Geometry: final body of the model. Coordinates: model frame, mm. A direction names the side the tool comes from. Give positions to 0.01 mm unless a question says otherwise; leave off trailing zeros. Order: outer loops, then holes, each group sorted by start corner. A loop starts at its lowest first (then second) coordinate and runs counter-clockwise, first axis right, second up. Notation, with made-up numbers: (-19, 36) - (7, 36) arc R26 cw to (7, 58) - close; hole circle Ø11 at (8.5, 11). An arc over 180 degrees is marked (long way). Use one line per item in the form item = value.
from build123d import *

# Parameters (mm, degrees)
SKETCH_1_W             = 300
SKETCH_1_H             = 300
EXTRUDE_2_DEPTH        = 5
SKETCH_4_W             = 45
SKETCH_4_H             = 60
CUT_EXTRUDE_3_DEPTH    = 5
SKETCH_5_OUTSIDE_W     = 386.858
SKETCH_5_OUTSIDE_H     = 386.858
SKETCH_5_OUTSIDE_W_2   = 250
SKETCH_5_OUTSIDE_H_2   = 300
CUT_EXTRUDE_4_DEPTH    = 5
SKETCH_6_R             = 1.75
SKETCH_6_R_2           = 1.25
CUT_EXTRUDE_5_DEPTH    = 5
SKETCH_7_W             = 50
SKETCH_7_H             = 70
CUT_EXTRUDE_6_DEPTH    = 10
SKETCH_8_W             = 30
SKETCH_8_H             = 24.494897428
SKETCH_8_W_2           = 120
SKETCH_8_H_2           = 10
CUT_EXTRUDE_7_DEPTH    = 10
FILLET_1_R             = 3
HOLE_WIZARD_M3_1_D     = 2.5
HOLE_WIZARD_M3_1_DEPTH = 10
HOLE_WIZARD_M3_1_TIP   = 0.751075774


with BuildPart() as part:
    # 草图1 → 凸台-拉伸2 (new body)
    with BuildSketch(Plane.XY):
        Rectangle(SKETCH_1_W, SKETCH_1_H)
    extrude(amount=EXTRUDE_2_DEPTH)

    # 草图4 → 切除-拉伸3 (cut)
    with BuildSketch(Plane.XY.offset(5)):
        with Locations((0, 120)):
            Rectangle(SKETCH_4_W, SKETCH_4_H)
    extrude(amount=-CUT_EXTRUDE_3_DEPTH, mode=Mode.SUBTRACT)

    # 草图5 outside → 切除-拉伸4 (cut)
    with BuildSketch(Plane.XY.offset(5)):
        Rectangle(SKETCH_5_OUTSIDE_W, SKETCH_5_OUTSIDE_H)
        Rectangle(SKETCH_5_OUTSIDE_W_2, SKETCH_5_OUTSIDE_H_2, mode=Mode.SUBTRACT)
    extrude(amount=-CUT_EXTRUDE_4_DEPTH, mode=Mode.SUBTRACT)

    # 草图6 → 切除-拉伸5 (cut)
    with BuildSketch(Plane.XY.offset(5)):
        with Locations((-85, 110)):
            Circle(SKETCH_6_R)
        with Locations((-61, 110)):
            Circle(SKETCH_6_R)
        with Locations((-61, 80)):
            Circle(SKETCH_6_R)
        with Locations((-85, 80)):
            Circle(SKETCH_6_R)
        with Locations((85, 80)):
            Circle(SKETCH_6_R)
        with Locations((61, 80)):
            Circle(SKETCH_6_R)
        with Locations((61, 110)):
            Circle(SKETCH_6_R)
        with Locations((85, 110)):
            Circle(SKETCH_6_R)
        with Locations((-47, -100)):
            Circle(SKETCH_6_R_2)
        with Locations((-47, -44)):
            Circle(SKETCH_6_R_2)
        with Locations((47, -44)):
            Circle(SKETCH_6_R_2)
        with Locations((47, -100)):
            Circle(SKETCH_6_R_2)
        with Locations((-35, 105)):
            Circle(SKETCH_6_R)
        with Locations((-35, 85)):
            Circle(SKETCH_6_R)
        with Locations((35, 85)):
            Circle(SKETCH_6_R)
        with Locations((35, 105)):
            Circle(SKETCH_6_R)
    extrude(amount=-CUT_EXTRUDE_5_DEPTH, mode=Mode.SUBTRACT)

    # 草图7 → 切除-拉伸6 (cut)
    with BuildSketch(Plane.XY.offset(5)):
        with Locations((-125, 95)):
            Rectangle(SKETCH_7_W, SKETCH_7_H)
        with Locations((125, 95)):
            Rectangle(SKETCH_7_W, SKETCH_7_H)
    extrude(amount=-CUT_EXTRUDE_6_DEPTH, mode=Mode.SUBTRACT)

    # 草图8 → 切除-拉伸7 (cut)
    with BuildSketch(Plane.XY.offset(5)):
        Polygon((-125, 130), (-73.75, 150), (-125, 150), align=None)
        Polygon((125, 130), (73.75, 150), (125, 150), align=None)
        with BuildLine():
            Line((75, -150), (125, -150))
            Line((125, -150), (125, 60))
            Line((125, 60), (105, 60))
            Line((105, 60), (105, -134.641016151))
            ThreePointArc((105, -134.641016151), (103.660254038, -139.641016151), (100, -143.301270189))
            ThreePointArc((100, -143.301270189), (87.940952255, -148.296291314), (75, -150))
        make_face()
        with Locations((-55, -137.752551286)):
            Rectangle(SKETCH_8_W, SKETCH_8_H)
        with Locations((55, -137.752551286)):
            Rectangle(SKETCH_8_W, SKETCH_8_H)
        with Locations((0, 145)):
            Rectangle(SKETCH_8_W_2, SKETCH_8_H_2)
        with BuildLine():
            Line((-105, 60), (-105, -134.641016151))
            ThreePointArc((-105, -134.641016151), (-103.660254038, -139.641016151), (-100, -143.301270189))
            ThreePointArc((-100, -143.301270189), (-87.940952255, -148.296291314), (-75, -150))
            Line((-75, -150), (-125, -150))
            Line((-125, -150), (-125, 60))
            Line((-125, 60), (-105, 60))
        make_face()
        with BuildLine():
            Line((-15.032646415, -7.416105565), (-8.618717278, -7.416105565))
            Line((-8.618717278, -7.416105565), (-8.618717278, -25.054410692))
            Line((-8.618717278, -25.054410692), (-15.032646415, -25.054410692))
            ThreePointArc((-15.032646415, -25.054410692), (-23.851798978, -16.235258128), (-15.032646415, -7.416105565))
        make_face()
        with BuildLine():
            Line((8.618717278, -25.054410692), (15.032646415, -25.054410692))
            ThreePointArc((15.032646415, -25.054410692), (23.851798978, -16.235258128), (15.032646415, -7.416105565))
            Line((15.032646415, -7.416105565), (8.618717278, -7.416105565))
            Line((8.618717278, -7.416105565), (8.618717278, -25.054410692))
        make_face()
        with BuildLine():
            ThreePointArc((-49.706822203, 9.446585999), (-68.824680462, -27.637553869), (-65.047087709, -69.188194384))
            ThreePointArc((-65.047087709, -69.188194384), (-58.959639066, -71.844151136), (-56.303682313, -65.756702493))
            ThreePointArc((-56.303682313, -65.756702493), (-59.605793483, -29.435996915), (-42.894279713, 2.980401704))
            ThreePointArc((-42.894279713, 2.980401704), (-43.06745881, 9.619765097), (-49.706822203, 9.446585999))
        make_face()
        with BuildLine():
            ThreePointArc((49.706822203, 9.446585999), (68.824680462, -27.637553869), (65.047087709, -69.188194384))
            ThreePointArc((65.047087709, -69.188194384), (58.959639066, -71.844151136), (56.303682313, -65.756702493))
            ThreePointArc((56.303682313, -65.756702493), (59.605793483, -29.435996915), (42.894279713, 2.980401704))
            ThreePointArc((42.894279713, 2.980401704), (43.06745881, 9.619765097), (49.706822203, 9.446585999))
        make_face()
    extrude(amount=-CUT_EXTRUDE_7_DEPTH, mode=Mode.SUBTRACT)

    # 圆角1
    fillet_1_edges = [part.edges().sort_by_distance(p)[0] for p in [
        (125, 130, 2.5),
        (-125, 130, 2.5),
        (-105, 60, 2.5),
        (105, 60, 2.5),
        (-40, -125.505102572, 2.5),
        (-40, -150, 2.5),
        (-70, -125.505102572, 2.5),
        (40, -150, 2.5),
        (40, -125.505102572, 2.5),
        (70, -125.505102572, 2.5),
    ]]
    fillet(fillet_1_edges, radius=FILLET_1_R)

    # M3 螺纹孔1
    with Locations(Plane.XY.offset(5)):
        with Locations((-30, -146), (30, -146), (30, -111), (-30, -111)):
            Hole(HOLE_WIZARD_M3_1_D / 2, depth=HOLE_WIZARD_M3_1_DEPTH)
            with Locations((0, 0, -(HOLE_WIZARD_M3_1_DEPTH + HOLE_WIZARD_M3_1_TIP / 2))):  # 118° drill point
                Cone(0, HOLE_WIZARD_M3_1_D / 2, HOLE_WIZARD_M3_1_TIP, mode=Mode.SUBTRACT)


solid = part.part
(1) Contact query for flat-ended pins moving along their axis: pin 1 Ø3 at (x, y) = (-35, 105) entering from -Z; pin 2 Ø2.5 at (x, z) = (-8, 3) entering from +Y; pin 3 Ø1.5 at (y, z) = (-72, 2) entering from -X; pin 4 Ø2.5 at (y, z) = (104, 2.5) entering from -X. Output: stop coordinate, or through.
Computed values:
pin_1 = through
pin_2 = 90
pin_3 = -105
pin_4 = -100
(2) Ray query, line 1 along X through (y, z) = (-111, 3.15); line 2 along Y through (x, z) = (30, 3.95); line 3 along X through (y, z) = (110, 2.2). Return the intervals inside material, ascending.
Computed values:
line_1 = -105 to -31.25, -28.75 to 28.75, 31.25 to 105
line_2 = -150 to -147.25, -144.75 to -112.25, -109.75 to 140
line_3 = -100 to -86.75, -83.25 to -62.75, -59.25 to -22.5, 22.5 to 59.25, 62.75 to 83.25, 86.75 to 100
(3) Cut plane A-A on y = 98. Output: boundary loops of the cut face in (x, z).
Computed values:
outline = (-100, 0) - (-22.5, 0) - (-22.5, 5) - (-100, 5) - close; (22.5, 0) - (100, 0) - (100, 5) - (22.5, 5) - close
(4) Cut plane C-C on z = 4.05. Give the number of separate pieces and of enclosed holes in the cut face, plus the area to 3 significant figures.
Computed values:
separate_pieces = 1
enclosed_holes = 24
area = 54,600 mm²
(5) Pull-direction query (Y, two-part tool) for faces 3 (the face through (-2, 2, 0)), 4 (the face through (88.12, -148.25, 2.54)), 5 (the face through (-23.85, -16.43, 2.54)); classes: released by +Y, released by -Y, zero draft, split by the parting line, or undercut.
Computed values:
face_3 = zero draft
face_4 = released by -Y
face_5 = undercut
(6) Reachability of faces 1 (the face through (-59.703, -29.944, 2.535)), 2 (the face through (92.2, 142.8, 2.5)) from +Z, -Z, +X, -X, +Y, -Y: full face, straight path, thin tool, end or side. Return the list, or none.
Computed values:
face_1 = +Z, -Z
face_2 = +Z, -Z, +X, +Y
(7) Cut plane B-B on y = -81.5. Output: boundary loops of the cut face in (x, z).
Computed values:
outline = (-105, 0) - (105, 0) - (105, 5) - (-105, 5) - close
